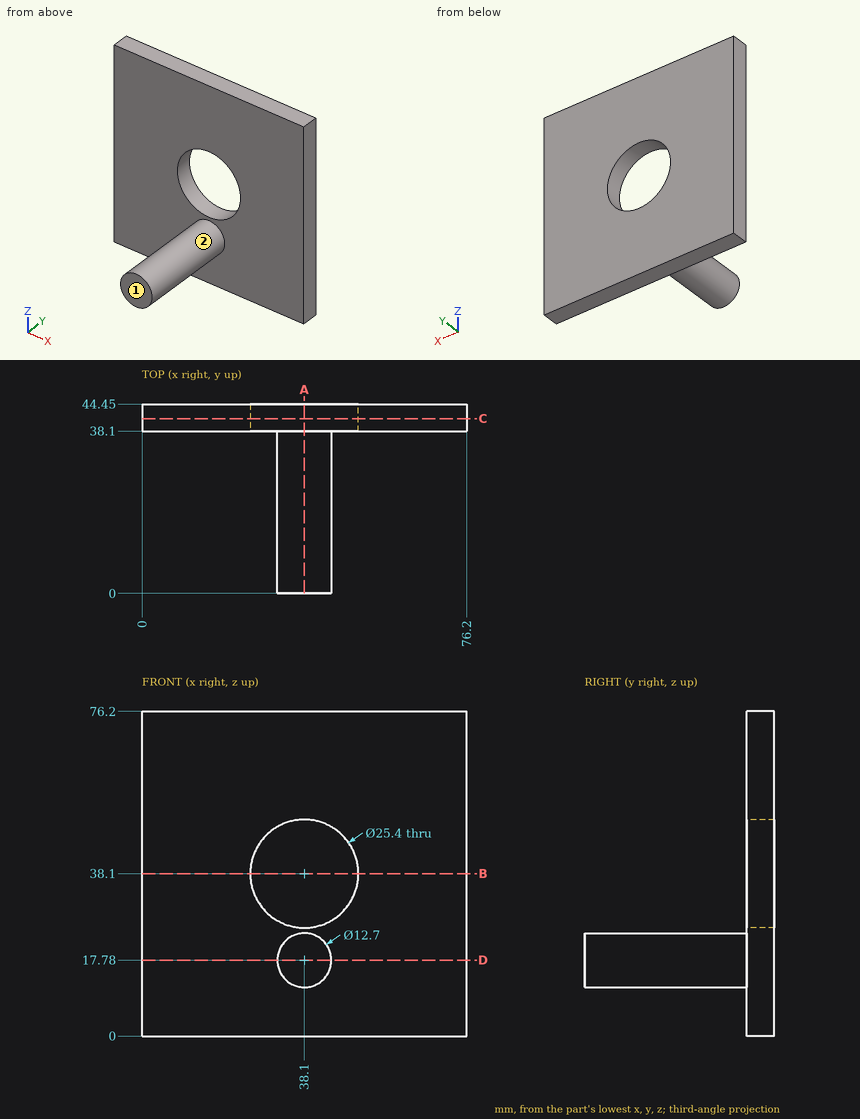
Check sheet for the drawn part. Datum: minimum x, y, z corner. Units: mm. A direction names the side the tool comes from. Round coordinates to 2 decimals unless told otherwise and drop trailing zeros. Loops run counter-clockwise (first coordinate to the right, second up) from the corner with the lowest first, then second, coordinate; pieces in that order, holes last. Notation, with made-up numbers: (-24.5, -15) -> (22.5, -15) arc R26 cw to (22.5, 19) -> close; hole circle Ø3 at (-23, 67). An arc over 180 degrees is marked (long way). Put each result on its own line as item: value. Start each with the question number.
1. Section check C-C (y = 41). Enter the section's corners in (x, z).
2. Access from +Z, -Z, +X, -X, +Y, -Y to the whole of each face (thin tool, end or side, straight path). Record for the marked faces 1 and 2.
3. Scan lines: probe 1 along Z at (x, y) = (38, 39); probe 2 along Y at (x, z) = (6, 20). Record each from-to range of solid material in increasing order.
4. Gauge pin test, flat ends, axial feed: pin 1 (12 mm diameter, centred on x = 19.5, z = 15.5, fed in from -Y); pin 2 (6 mm diameter, centred on y = 5, z = 23, fed in from -X); pin 3 (15 mm diameter, centred on x = 38.1, z = 38.1, fed in from +Y). Record the tip position at first contact, or that the pin passes through.
5. Section check B-B (z = 38.1). Enter the section's corners in (x, y).
6. Section check D-D (z = 17.78). Enter the section's corners in (x, y), plus the area to 3 significant figures.
7. Section check A-A (x = 38.1). Enter the section's corners in (y, z), plus the area to 3 significant figures.
Findings:
1. outline: (0, 0) -> (76.2, 0) -> (76.2, 76.2) -> (0, 76.2) -> close; hole circle Ø25.4 at (38.1, 38.1)
2. face 1: +Z, -Z, +X, -X, -Y
2. face 2: -Y
3. probe 1: z = 0 to 25.4, 50.8 to 76.2
3. probe 2: y = 38.1 to 44.45
4. pin 1: stops at y = 38.1
4. pin 2: stops at x = 32.15
4. pin 3: passes through
5. outline: (0, 38.1) -> (25.4, 38.1) -> (25.4, 44.45) -> (0, 44.45) -> close; (50.8, 38.1) -> (76.2, 38.1) -> (76.2, 44.45) -> (50.8, 44.45) -> close
6. outline: (0, 38.1) -> (31.75, 38.1) -> (31.75, 0) -> (44.45, 0) -> (44.45, 38.1) -> (76.2, 38.1) -> (76.2, 44.45) -> (0, 44.45) -> close
6. area: 968 mm^2
7. outline: (0, 11.43) -> (38.1, 11.43) -> (38.1, 0) -> (44.45, 0) -> (44.45, 25.4) -> (38.1, 25.4) -> (38.1, 24.13) -> (0, 24.13) -> close; (38.1, 50.8) -> (44.45, 50.8) -> (44.45, 76.2) -> (38.1, 76.2) -> close
7. area: 806 mm^2
